```python
from build123d import *

# Parameters (mm, degrees)
SKETCH1_R              = 31
BASE_EXTRUDE_DEPTH     = 12
M10_GEVINDHULLER_D     = 8.5
M10_GEVINDHULLER_DEPTH = 24
M10_GEVINDHULLER_TIP   = 2.553657631
SKETCH7_R              = 7.125
F_14_25_HULLER_DEPTH   = 25


with BuildPart() as part:
    # Sketch1 → Base-Extrude (new body, symmetric)
    with BuildSketch(Plane.XY):
        with BuildLine():
            Line((34, 46), (21.540659229, 46))
            ThreePointArc((21.540659229, 46), (19.71491737, 46.168079197), (17.950549357, 46.666666667))
            ThreePointArc((17.950549357, 46.666666667), (0, 50), (-17.950549357, 46.666666667))
            ThreePointArc((-17.950549357, 46.666666667), (-19.71491737, 46.168079197), (-21.540659229, 46))
            Line((-21.540659229, 46), (-34, 46))
            ThreePointArc((-34, 46), (-42.485281374, 42.485281374), (-46, 34))
            Line((-46, 34), (-46, 0))
            Line((-46, 0), (-46, -33.587572106))
            ThreePointArc((-46, -33.587572106), (-42.364484041, -42.364484041), (-33.587572106, -46))
            Line((-33.587572106, -46), (-20.784609691, -46))
            ThreePointArc((-20.784609691, -46), (-15.784609691, -47.339745962), (-12.124355653, -51))
            Line((-12.124355653, -51), (-8.660254038, -57))
            ThreePointArc((-8.660254038, -57), (0, -62), (8.660254038, -57))
            Line((8.660254038, -57), (12.124355653, -51))
            ThreePointArc((12.124355653, -51), (15.784609691, -47.339745962), (20.784609691, -46))
            Line((20.784609691, -46), (25.502525317, -46))
            ThreePointArc((25.502525317, -46), (35.069611126, -47.903011687), (43.180194847, -53.32233047))
            Line((43.180194847, -53.32233047), (48.928932188, -59.071067812))
            ThreePointArc((48.928932188, -59.071067812), (61.735764364, -60.191520443), (65.06307787, -47.773817383))
            Line((65.06307787, -47.773817383), (48.810766389, -12.920622936))
            ThreePointArc((48.810766389, -12.920622936), (46.711119786, -6.735263502), (46, -0.242075084))
            Line((46, -0.242075084), (46, 34))
            ThreePointArc((46, 34), (42.485281374, 42.485281374), (34, 46))
        make_face()
        Circle(SKETCH1_R, mode=Mode.SUBTRACT)
    extrude(amount=BASE_EXTRUDE_DEPTH, both=True)

    # Sketch2 → Uddrejning (revolve, cut)
    with BuildSketch(Plane(origin=(0, 0, 0), x_dir=(0, 0, -1), z_dir=(1, 0, 0))):
        Polygon((12, 38.5), (5, 38.5), (5, 35), (-12, 35), (-12, 0), (12, 0), align=None)
    revolve(axis=Axis((0, 0, 0), (0, 0, -1)), mode=Mode.SUBTRACT)

    # M10 gevindhuller
    with Locations(Plane.XY.offset(12)):
        with Locations((56, -52), (0, -52)):
            Hole(M10_GEVINDHULLER_D / 2, depth=M10_GEVINDHULLER_DEPTH)
            with Locations((0, 0, -(M10_GEVINDHULLER_DEPTH + M10_GEVINDHULLER_TIP / 2))):  # 118° drill point
                Cone(0, M10_GEVINDHULLER_D / 2, M10_GEVINDHULLER_TIP, mode=Mode.SUBTRACT)

    # Sketch7 → ø14.25 huller (cut, through all)
    with BuildSketch(Plane.XY.offset(12)):
        with Locations((33.587572106, 33.587572106)):
            Circle(SKETCH7_R)
        with Locations((33.587572106, -33.587572106)):
            Circle(SKETCH7_R)
        with Locations((-33.587572106, -33.587572106)):
            Circle(SKETCH7_R)
        with Locations((-33.587572106, 33.587572106)):
            Circle(SKETCH7_R)
    extrude(amount=-F_14_25_HULLER_DEPTH, mode=Mode.SUBTRACT)


solid = part.part
```
The listing builds one solid part. Answer for the finished solid, in the listing's coordinates (mm). A direction names the side the tool comes from. Round coordinates to 2 decimals unless told otherwise and drop trailing zeros. Loops run counter-clockwise (first coordinate to the right, second up) from the corner with the lowest first, then second, coordinate; pieces in that order, holes last. Notation, with made-up numbers: (80.25, -9.5) - (101.25, -9.5) arc R16 cw to (101.25, 16.5) - close; hole circle Ø3 at (55, -27). An arc over 180 degrees is marked (long way). Return JSON: item names as keys, results as strings. Group by question number.
1. The part is cut by section B-B on y = -17.5. Determine the outline of the cut face in (x, z).
2. The part is cut by section C-C on x = 56. Determine the outline of the cut face in (y, z), then the cut area to 3 significant figures.
3. The mould has two halves that part along Y. Classify faces 6 (the cylindrical face through (34.94, -47.85, 0.17)), 7 (the flat face through (-34, -9, -5)), 8 (the flat face through (28, 46, 0)), 9 (the cylindrical face through (54.04, -55.77, -0.17)): pulls with the +Y half, pulls with the -Y half, needs draft (parallel to the pull), parting line crosses it, or undercut.
4. Consider probe 1 along X at (y, z) = (0, -10.5); probe 2 along X at (y, z) = (-52, 6.5); probe 3 along Y at (x, z) = (39, 1.25). Determine where each line is inside the solid, lowest interval first.
5. The part is cut by section A-A on x = 0. Determine the outline of the cut face in (y, z), then the cut area to 3 significant figures.
6. The part is cut by section D-D on z = -7.25. State how many separate pieces and enclosed holes the cut face has, then the cut area to 3 significant figures.
7. Each of these flat-tipped pins is pushed along its axis until it touches: P1, Ø8, axis at x = 45.5, z = 1, coming from the -Y side; P2, Ø12, axis at y = 31.5, z = -6.5, coming from the +X side; P3, Ø3.5, axis at x = -26.5, z = 0, coming from the +Y side. Where does it stop, or does it pass through?
8. Which of the six approach directions +Z, -Z, +X, -X, +Y, -Y give full straight-line access (tool end or side, diameter ignored) to faces 1 (the flat face through (-28, 46, 0)), 2 (the cylindrical face through (15.721, -47.377, 0.168)), 3 (the cylindrical face through (0.92, -56.15, -0.17)), 4 (the cylindrical face through (-15.848, -47.303, 0.168)), 5 (the cylindrical face through (-23.43, -30.55, -8.45))?
Resolved:
{
 "1": {"outline": "(-46, -12) - (-34.29, -12) - (-34.29, -5) - (-30.31, -5) - (-30.31, 12) - (-46, 12) - close; (30.31, -5) - (34.29, -5) - (34.29, -12) - (50.95, -12) - (50.95, 12) - (30.31, 12) - close"},
 "2": {"outline": "(-62, -12) - (-56.25, -12) - (-56.25, 12) - (-62, 12) - close; (-47.75, -12) - (-28.34, -12) - (-28.34, 12) - (-47.75, 12) - close", "area": "604 mm²"},
 "3": {"face 6": "pulls with the -Y half", "face 7": "undercut", "face 8": "pulls with the +Y half", "face 9": "undercut"},
 "4": {"probe 1": "x = -46 to -38.5, 38.5 to 46", "probe 2": "x = -11.55 to -4.25, 4.25 to 11.55, 41.75 to 51.75, 60.25 to 66", "probe 3": "y = -49.96 to -38.22, -28.95 to 28.95, 38.22 to 44.91"},
 "5": {"outline": "(-62, -12) - (-56.25, -12) - (-56.25, 12) - (-62, 12) - close; (-47.75, -12) - (-38.5, -12) - (-38.5, -5) - (-35, -5) - (-35, 12) - (-47.75, 12) - close; (35, -5) - (38.5, -5) - (38.5, -12) - (50, -12) - (50, 12) - (35, 12) - close", "area": "755 mm²"},
 "6": {"separate pieces": "1", "enclosed holes": "7", "area": "4,100 mm²"},
 "7": {"P1": "stops at y = -59.6", "P2": "stops at x = 46", "P3": "stops at y = 46"},
 "8": {"face 1": "+Z, -Z, -X, +Y", "face 2": "+Z, -Z, -Y", "face 3": "+Z, -Z", "face 4": "+Z, -Z, -X, -Y", "face 5": "-Z"}
}
